Could you check a few things on this model? Use its own coordinates, in mm. A direction names the side the tool comes from. Round coordinates to 2 decimals unless told otherwise and drop trailing zeros. Loops run counter-clockwise (first coordinate to the right, second up) from the corner with the lowest first, then second, coordinate; pieces in that order, holes last. Notation, with made-up numbers: M 7.5,37.5 L 31.5,37.5 A25 cw 31.5,74.5 Z; hole C 34.25,-27.75 d6. An arc over 180 degrees is marked long. Answer in a Markdown table with one row per item.
```python
from build123d import *

# Parameters (mm, degrees)
F0_R     = 20
F1_DEPTH = 53
F0_R_2   = 22.5
F2_DEPTH = 2
F3_T     = -2.5
F4_DEPTH = 3
F5_SIZE  = 1
F7_R     = 2


# Not quite as in the source:
# - a fillet or chamfer that OpenCascade refuses, or shapes differently, is made with other operations: its cross-section is extruded or revolved along the edge and cut away or added


with BuildPart() as f1:
    # F0 (on Top) → F1 (new body)
    with BuildSketch(Plane.XY):
        Circle(F0_R)
    extrude(amount=F1_DEPTH)

    # F0 (on Top) → F2 (join)
    with BuildSketch(Plane.XY):
        Circle(F0_R_2)
        Circle(F0_R, mode=Mode.SUBTRACT)
    extrude(amount=F2_DEPTH)

    # F3
    f3_openings = [f1.faces().sort_by_distance(p)[0] for p in [
        (0, 0, 53),
    ]]
    offset(amount=F3_T, openings=f3_openings)

    # F4 (cut): a face of the model
    f4_faces = [f1.faces().sort_by_distance(p)[0] for p in [
        (0, 0, 2.5),
    ]]
    extrude(f4_faces, amount=-F4_DEPTH, mode=Mode.SUBTRACT)

    # F5
    f5_edges = [f1.edges().sort_by_distance(p)[0] for p in [
        (-20, 0, 53),
    ]]
    chamfer(f5_edges, length=F5_SIZE)

    # F6: fillet of radius 2 on 2 edges, made by hand

    # F6_s1 → F6_t2 (revolve, cut)
    with BuildSketch(Plane.XZ):
        with BuildLine():
            ThreePointArc((19, 53), (17.9188611699, 52.2882531983), (17.5, 51.0635083269))
            Line((17.5, 51.0635083269), (17.5, 53))
            Line((17.5, 53), (19, 53))
        make_face()
    revolve(axis=Axis((0, 0, 53), (0, 0, 1)), mode=Mode.SUBTRACT)

    # F7
    f7_edges = [f1.edges().sort_by_distance(p)[0] for p in [
        (-17.5, 0, 0),
    ]]
    fillet(f7_edges, radius=F7_R)


solid = f1.part
```
1) I need wall thicknesses on line 1 (Y direction, x = 0.5, z = 40.5); line 2 (X direction, y = 14.5, z = 17); line 3 (X direction, y = 12, z = 42). Which ranges of each line are inside material? Lowest first, please.
Computed:
| item | result |
|---|---|
| line 1 | y = -19.99 to -17.49, 17.49 to 19.99 |
| line 2 | x = -13.77 to -9.8, 9.8 to 13.77 |
| line 3 | x = -16 to -12.74, 12.74 to 16 |
2) Will these pins go through, and if not, where does the flat tip stop? P1, Ø12, axis at x = 12.5, z = 14.5, coming from the -Y side; P2, Ø6, axis at x = -16.5, z = 23, coming from the +Y side; P3, Ø6, axis at y = -12.5, z = 9.5, coming from the -X side.
Computed:
| item | result |
|---|---|
| P1 | stops at y = -18.91 |
| P2 | stops at y = 14.76 |
| P3 | stops at x = -17.6 |
3) I want a section at A-A, the plane y = 0. Please give me the cut outline in (x, z), plus the area to 3 significant figures.
Computed:
| item | result |
|---|---|
| outline | M -22.5,0 L -19.5,0 A2 ccw -17.5,2 L -17.5,51.06 A2 ccw -19,53 L -20,52 L -20,2 L -22.5,2 Z; M 17.5,2 A2 ccw 19.5,0 L 22.5,0 L 22.5,2 L 20,2 L 20,52 L 19,53 A2 ccw 17.5,51.06 Z |
| area | 271 mm² |
4) Which directions (+Z, -Z, +X, -X, +Y, -Y) give clear straight access to the entire face, cutting with the end or side of a thin tool? Please do faces 1 (the face through (-20.1, -1.6, 2)), 2 (the face through (10.382, -19.961, 0.986)).
Computed:
| item | result |
|---|---|
| face 1 | +Z |
| face 2 | +Z, -Z |
5) I want a section at C-C, the plane z = 3. Please give me the cut outline in (x, y), plus the area to 3 significant figures.
Computed:
| item | result |
|---|---|
| outline | C 0,0 d40; hole C 0,0 d35 |
| area | 295 mm² |
